The drawing under review shows one solid part. Ordinate dimensions are in mm from its lowest x, y, z. A direction names the side the tool comes from. Coordinates: 2 decimals unless noted, no trailing zeros. Order: outer loops, then holes, each group sorted by start corner. A loop starts at its lowest first (then second) coordinate and runs counter-clockwise, first axis right, second up.
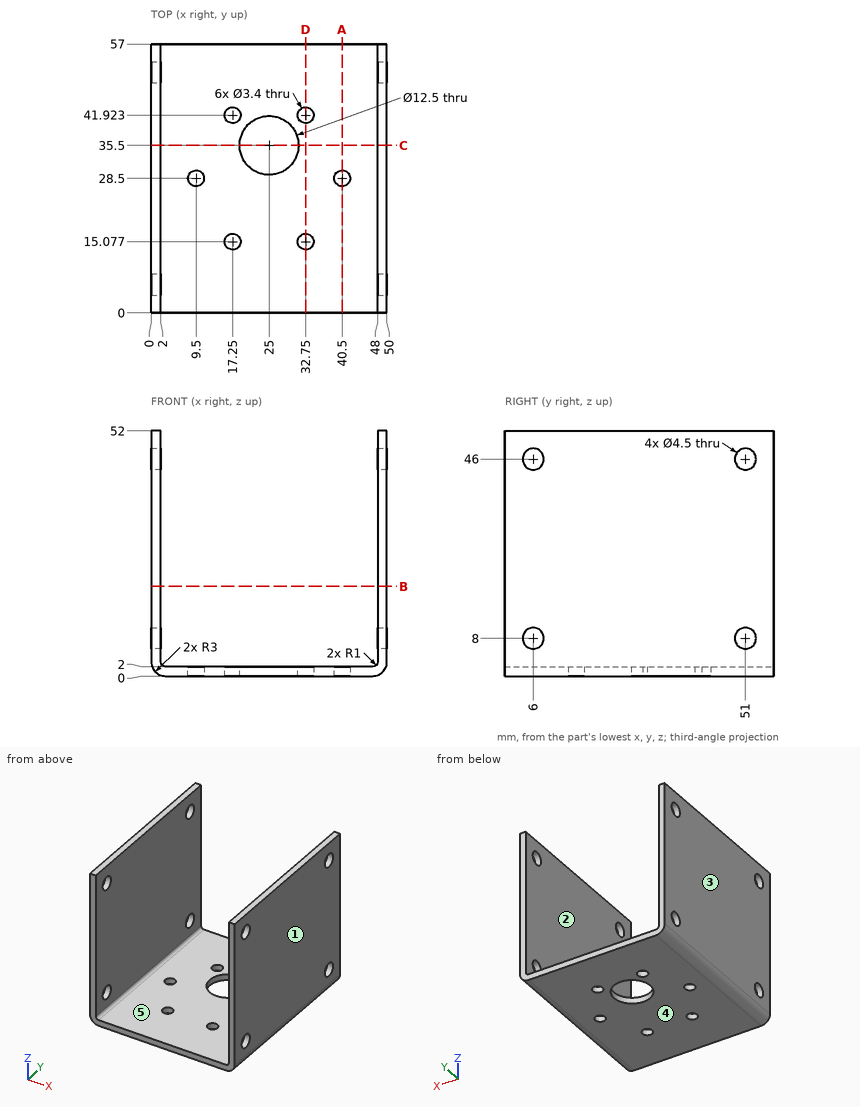
1. Machinability: for the marked faces 1 and 2, which of the approach directions +Z, -Z, +X, -X, +Y, -Y give a long, thin tool a straight path to every point of the face, cutting with its end or side? Answer none if there is none.
Answer below:
face 1: +Z, -Z, +X, +Y, -Y
face 2: +Z, +Y, -Y
2. Take a section at C-C, the plane y = 35.5. Give the boundary of the cut face in (x, z).
Answer below:
outline: (0, 3) arc R3 ccw to (3, 0) - (18.75, 0) - (18.75, 2) - (3, 2) arc R1 cw to (2, 3) - (2, 52) - (0, 52) - close; (31.25, 0) - (47, 0) arc R3 ccw to (50, 3) - (50, 52) - (48, 52) - (48, 3) arc R1 cw to (47, 2) - (31.25, 2) - close
3. Take a section at B-B, the plane z = 19. Give the boundary of the cut face in (x, y), plus the area to 3 significant figures.
Answer below:
outline: (0, 0) - (2, 0) - (2, 57) - (0, 57) - close; (48, 0) - (50, 0) - (50, 57) - (48, 57) - close
area: 228 mm2
4. The part is to be moulded in two halves that separate along Z. For the marked faces 3, 4 and 5, say which applies: +Z half, -Z half, draft (parallel to the pull), parting line (faces both ways), or undercut.
Answer below:
face 3: draft
face 4: -Z half
face 5: +Z half
5. Take a section at A-A, the plane x = 40.5. Give the boundary of the cut face in (y, z).
Answer below:
outline: (0, 0) - (26.8, 0) - (26.8, 2) - (0, 2) - close; (30.2, 0) - (57, 0) - (57, 2) - (30.2, 2) - close
6. Clearance check with flat-ended pins moving along their axes: pin 1 Ø4 at (x, y) = (40.5, 28.5) entering from +Z; pin 2 Ø4 at (y, z) = (6, 8) entering from +X. State where each tip first meets the part, or that it passes through.
Answer below:
pin 1: stops at z = 2
pin 2: passes through
7. Take a section at D-D, the plane x = 32.75. Give the boundary of the cut face in (y, z), plus the area to 3 significant figures.
Answer below:
outline: (0, 0) - (13.38, 0) - (13.38, 2) - (0, 2) - close; (16.78, 0) - (40.22, 0) - (40.22, 2) - (16.78, 2) - close; (43.62, 0) - (57, 0) - (57, 2) - (43.62, 2) - close
area: 100 mm2
8. To check wall thickness, follow L1, parallel to Y at x = 1.3, z = 8; L2, parallel to Y at x = 32.75, z = 0.8; L3, parallel to X at y = 29, z = 35.5. State the ranges of each line that lie inside material, in increasing order.
Answer below:
L1: y = 0 to 3.75, 8.25 to 48.75, 53.25 to 57
L2: y = 0 to 13.38, 16.78 to 40.22, 43.62 to 57
L3: x = 0 to 2, 48 to 50
